Check sheet for the modelled part. Datum: model origin and axes. Units: mm. A direction names the side the tool comes from. Round coordinates to 2 decimals unless told otherwise and drop trailing zeros. Loops run counter-clockwise (first coordinate to the right, second up) from the corner with the lowest first, then second, coordinate; pieces in that order, holes last. Notation, with made-up numbers: (-6.5, 60.5) -> (15.5, 60.5) arc R8 cw to (15.5, 65.5) -> close; hole circle Ø3 at (39, 62.25). An arc over 180 degrees is marked (long way). Return JSON: item names as keys, results as strings.
from build123d import *

# Parameters (mm, degrees)
SKETCH1_R           = 14
SKETCH1_W           = 4.7625
SKETCH1_H           = 4.7625
BOSS_EXTRUDE1_DEPTH = 12.7
CUT_EXTRUDE2_DEPTH  = 12.7
CIRPATTERN1_COUNT   = 12
CUT_EXTRUDE3_DEPTH  = 12.7
BOSS_EXTRUDE2_DEPTH = 12.7


with BuildPart() as part:
    # Sketch1 → Boss-Extrude1 (new body)
    with BuildSketch(Plane.XY):
        Circle(SKETCH1_R)
        Rectangle(SKETCH1_W, SKETCH1_H, mode=Mode.SUBTRACT)
    extrude(amount=BOSS_EXTRUDE1_DEPTH)

    # Sketch2 → Cut-Extrude2 (cut)
    with BuildSketch(Plane.XY.offset(12.7)):
        with BuildLine():
            Line((9.765735466, 5.63825), (8.425772987, 4.386040421))
            ThreePointArc((8.425772987, 4.386040421), (8.775931679, 3.635109924), (9.05932014, 2.856522291))
            Line((9.05932014, 2.856522291), (10.89226258, 2.918572962))
            add(Edge.make_bspline(
                [(10.89226258, 2.918572962), (10.926225774, 2.926110483), (11.022290818, 2.942700204), (11.208093043, 2.95599604), (11.510593122, 2.951165366), (11.900233077, 2.905990048), (12.393614042, 2.803046766), (12.953297572, 2.62879349), (13.387020142, 2.449311198), (13.697491187, 2.299105356), (13.848549614, 2.220883572)],
                knots=[0, 0, 0, 0, 0, 0.005604071, 0.015718253, 0.029959921, 0.048733673, 0.068727069, 0.096888899, 0.124316379, 0.124316379, 0.124316379, 0.124316379, 0.124316379], degree=4))
            ThreePointArc((13.848549614, 2.220883572), (12.957872383, 5.367326481), (11.362805176, 8.222001507))
            add(Edge.make_bspline(
                [(9.765735466, 5.63825), (9.795080903, 5.656935773), (9.874739851, 5.713133312), (10.01552344, 5.835113749), (10.226007495, 6.052429409), (10.469580775, 6.359890238), (10.745661909, 6.781555156), (11.018202255, 7.300526849), (11.197977279, 7.734128165), (11.311301892, 8.059875916), (11.362805176, 8.222001507)],
                knots=[0, 0, 0, 0, 0, 0.005604071, 0.015718253, 0.029959921, 0.048733673, 0.068727069, 0.096888899, 0.124316379, 0.124316379, 0.124316379, 0.124316379, 0.124316379], degree=4))
        make_face()
    cut_extrude2 = extrude(amount=-CUT_EXTRUDE2_DEPTH, mode=Mode.SUBTRACT)

    # CirPattern1: Cut-Extrude2 ×12 about axis
    cirpattern1_axis = Axis((0, 0, 12.7), (0, 0, -1))
    for i in range(1, CIRPATTERN1_COUNT):
        add(cut_extrude2.rotate(cirpattern1_axis, i * 360 / CIRPATTERN1_COUNT), mode=Mode.SUBTRACT)

    # Sketch4 → Cut-Extrude3 (cut)
    with BuildSketch(Plane.XY.offset(12.7)):
        with BuildLine():
            Line((-9.431447157, 1.130842839), (-13.900437961, 1.666680677))
            ThreePointArc((-13.900437961, 1.666680677), (-1.645492098, -13.902962122), (13.905453984, -1.624299696))
            Line((13.905453984, -1.624299696), (9.434850528, -1.102087344))
            ThreePointArc((9.434850528, -1.102087344), (-1.116466388, -9.4331598), (-9.431447157, 1.130842839))
        make_face()
    extrude(amount=-CUT_EXTRUDE3_DEPTH, mode=Mode.SUBTRACT)

    # Sketch5 → Boss-Extrude2 (add)
    with BuildSketch(Plane.XY.offset(12.7)):
        with BuildLine():
            Line((-13.086503174, 4.974277301), (-9.389446127, -1.445095645))
            Line((-9.389446127, -1.445095645), (-9.388388384, -1.445394253))
            ThreePointArc((-9.388388384, -1.445394253), (-9.484867836, -0.517960557), (-9.489953664, 0.414464066))
            ThreePointArc((-9.489953664, 0.414464066), (-9.417734738, 1.2398683), (-9.273862528, 2.055839199))
            Line((-9.273862528, 2.055839199), (-10.89226258, 2.918572962))
            add(Edge.make_bspline(
                [(-10.89226258, 2.918572962), (-10.925444329, 2.929026875), (-11.016933958, 2.962692277), (-11.184491323, 3.044078857), (-11.444048739, 3.199512383), (-11.75889918, 3.433455334), (-12.134707988, 3.769297313), (-12.526899585, 4.194215821), (-12.808483679, 4.559768992), (-12.998544728, 4.838012668), (-13.086503174, 4.974277301)],
                knots=[0, 0, 0, 0, 0, 0.005604071, 0.015718253, 0.029959921, 0.048733673, 0.068727069, 0.096888899, 0.123039083, 0.123039083, 0.123039083, 0.123039083, 0.123039083], degree=4))
        make_face()
    extrude(amount=-BOSS_EXTRUDE2_DEPTH)


solid = part.part
Q1. Go/stop test with flat-tipped pins: pin 1 (5 mm diameter, centred on y = 0.5, z = 3.5, fed in from -X); pin 2 (2 mm diameter, centred on y = 4, z = 6, fed in from +X); pin 3 (2 mm diameter, centred on x = -2.5, z = 10, fed in from +Y). Record where each tip stops, or that it passes through.
Results list:
{"pin 1": "x = -11.95", "pin 2": "x = 9.08", "pin 3": "y = 13.92"}
Q2. Section check B-B (x = -4.75). Record the boundary of the cut face in (y, z).
Results list:
{"outline": "(-8.23, 0) -> (8.82, 0) -> (8.82, 12.7) -> (-8.23, 12.7) -> close"}
Q3. Section check A-A (y = -7.5). Record the boundary of the cut face in (x, z), then the cut area to 3 significant figures.
Results list:
{"outline": "(-5.83, 0) -> (5.83, 0) -> (5.83, 12.7) -> (-5.83, 12.7) -> close", "area": "148 mm^2"}
Q4. Tool access check on faces 1 (the flat face through (-3, 2, 0)), 2 (the flat face through (7.18, 7.48, 6.44)), 3 (the cylindrical face through (-7.543, 5.773, 6.439)). Record the directions out of +Z, -Z, +X, -X, +Y, -Y that give a thin tool (end or side, any length) a straight path to the whole face; none if there is none.
Results list:
{"face 1": "-Z, +X, -X, +Y, -Y", "face 2": "+Z, -Z, +Y", "face 3": "+Z, -Z"}
Q5. Draft check along X on faces 4 (the flat face through (-8.901, 5.375, 6.439)), 5 (the flat face through (-7.48, 7.18, 6.44)), 6 (the flat face through (-3, 2, 12.7)). Enter one of: released by +X, released by -X, zero draft, split by the parting line, or undercut.
Results list:
{"face 4": "undercut", "face 5": "released by -X", "face 6": "zero draft"}
Q6. Material ranges on line 1 (Y direction, x = 1.25, z = 5); line 2 (X direction, y = -7, z = 2.5); line 3 (Y direction, x = 2.25, z = 2.75), recorded low to high.
Results list:
{"line 1": "-9.42 to -2.38, 2.38 to 9.42", "line 2": "-6.42 to 6.42", "line 3": "-9.23 to -2.38, 2.38 to 9.64"}
